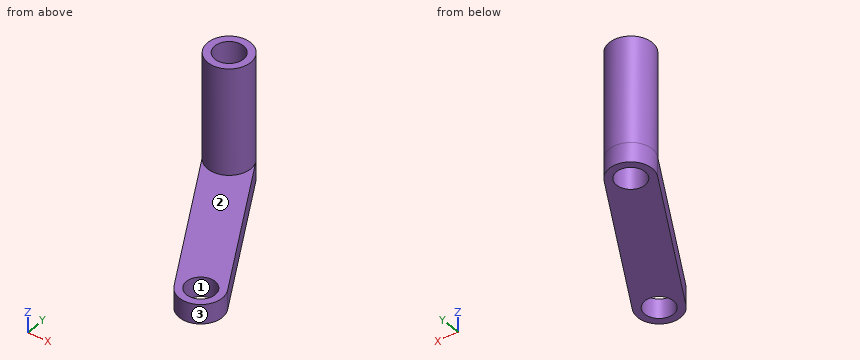
```python
from build123d import *

# Parameters (mm, degrees)
SKETCH1_R           = 2.2
BOSS_EXTRUDE1_DEPTH = 3
SKETCH2_R           = 3.3
SKETCH2_R_2         = 2.2
BOSS_EXTRUDE2_DEPTH = 16.4


with BuildPart() as part:
    # Sketch1 → Boss-Extrude1 (new body)
    with BuildSketch(Plane(origin=(0, 0, 0), x_dir=(-1, 0, 0), z_dir=(0, 0, 1))):
        with BuildLine():
            Line((26.852970862, 7.356194523), (39.052970862, -15.643805477))
            ThreePointArc((39.052970862, -15.643805477), (37.684063375, -20.105429878), (33.222438974, -18.736522391))
            Line((33.222438974, -18.736522391), (21.022438974, 4.263477609))
            ThreePointArc((21.022438974, 4.263477609), (22.391346461, 8.725102009), (26.852970862, 7.356194523))
        make_face()
        with Locations(Location((23.937704918, 5.809836066, 0), (0, 0, 180))):
            Circle(SKETCH1_R, mode=Mode.SUBTRACT)
        with Locations(Location((36.137704918, -17.190163934, 0), (0, 0, 180))):
            Circle(SKETCH1_R, mode=Mode.SUBTRACT)
    extrude(amount=BOSS_EXTRUDE1_DEPTH)

    # Sketch2 → Boss-Extrude2 (add)
    with BuildSketch(Plane.XY.offset(3)):
        with Locations(Location((-36.137704918, 17.190163934, 0), (0, 0, 207.943034423))):
            Circle(SKETCH2_R)
        with Locations((-36.137704918, 17.190163934)):
            Circle(SKETCH2_R_2, mode=Mode.SUBTRACT)
    extrude(amount=BOSS_EXTRUDE2_DEPTH)


solid = part.part
```
Check sheet for the modelled part. Datum: model origin and axes. Units: mm. Face numbers are marked on the shaded views. Coordinates: 2 decimals unless noted, no trailing zeros. Write each loop counter-clockwise with the first axis right and the second up, starting at its lowest first coordinate (ties: lowest second). Pieces come first, ordered by that corner, then holes. Notation, with made-up numbers: M 63,41 L 101,41 A33 cw 101,80 Z; hole C 37,86 d6. An arc over 180 degrees is marked long. Write item = value, one per line. Start each with the question number.
1. Mould release check, pull along Y, two halves, no side actions. Record for the marked faces 1, 2 and 3: pulls with the +Y half, pulls with the -Y half, needs draft (parallel to the pull), parting line crosses it, or undercut.
2. Go/stop test with flat-tipped pins: pin 1 (3 mm diameter, centred on y = 14.5, z = 10, fed in from -X); pin 2 (10 mm diameter, centred on y = 5, z = 2.5, fed in from +X); pin 3 (4 mm diameter, centred on y = 15.5, z = 7, fed in from +X). Record where each tip stops, or that it passes through.
3. Sectioned sample at C-C (z = 1.75). Record the cut outline in (x, y).
4. Sectioned sample at A-A (y = 18). Record the cut outline in (x, z).
5. Sectioned sample at B-B (x = -35.5). Record the cut outline in (y, z), then the cut area to 3 significant figures.
6. Thickness scan on probe 1 along Z at (x, y) = (-21.75, -3.25); probe 2 along Y at (x, z) = (-37.25, 6.5); probe 3 along Y at (x, z) = (-35.25, 7.25). Record the ranges inside material, lowest first.
7. Sectioned sample at D-D (z = 15). Record the cut outline in (x, y), then the cut area to 3 significant figures.
The answers:
q1.face_1 = undercut
q1.face_2 = needs draft
q1.face_3 = parting line crosses it
q2.pin_1 = -39.22
q2.pin_2 = -23.28
q2.pin_3 = -32.84
q3.outline = M -39.05,15.64 L -26.85,-7.36 A3.3 ccw -21.02,-4.26 L -33.22,18.74 A3.3 ccw Z; hole C -36.14,17.19 d4.4; hole C -23.94,-5.81 d4.4
q4.outline = M -39.34,0 L -38.18,0 L -38.18,19.4 L -39.34,19.4 Z; M -34.09,0 L -32.83,0 L -32.83,3 L -32.94,3 L -32.94,19.4 L -34.09,19.4 Z
q5.outline = M 8.95,0 L 15.08,0 L 15.08,19.4 L 13.95,19.4 L 13.95,3 L 8.95,3 Z; M 19.3,0 L 20.43,0 L 20.43,19.4 L 19.3,19.4 Z
q5.area = 59.0 mm²
q6.probe_1 = 0 to 3
q6.probe_2 = 14.08 to 15.29, 19.09 to 20.3
q6.probe_3 = 14.01 to 15.18, 19.2 to 20.37
q7.outline = C -36.14,17.19 d6.6; hole C -36.14,17.19 d4.4
q7.area = 19.0 mm²
